```python
from build123d import *

# Parameters (mm, degrees)
CROQUIS1_W              = 30
CROQUIS1_H              = 10
SALIENTE_EXTRUIR1_DEPTH = 2
CORTAR_EXTRUIR2_DEPTH   = 11
CROQUIS3_W              = 11.193843072
CROQUIS3_H              = 1
CROQUIS3_W_2            = 11.806156928
SALIENTE_EXTRUIR3_DEPTH = 1.5
CORTAR_EXTRUIR3_DEPTH   = 11.5
CROQUIS5_W              = 1.4
CROQUIS5_H              = 5
CORTAR_EXTRUIR4_DEPTH   = 10
CROQUIS6_W              = 8
CROQUIS6_H              = 5
SALIENTE_EXTRUIR4_DEPTH = 6
CROQUIS7_W              = 6.2
CROQUIS7_H              = 6
CORTAR_EXTRUIR5_DEPTH   = 11
CORTAR_EXTRUIR6_DEPTH   = 11
REDONDEO1_R             = 1
CROQUIS9_W              = 0.4
CROQUIS9_H              = 1
CORTAR_EXTRUIR7_DEPTH   = 23


with BuildPart() as part:
    # Croquis1 → Saliente-Extruir1 (new body)
    with BuildSketch(Plane.XY):
        Rectangle(CROQUIS1_W, CROQUIS1_H)
    extrude(amount=SALIENTE_EXTRUIR1_DEPTH)

    # Croquis2 → Cortar-Extruir2 (cut)
    with BuildSketch(Plane.XY.offset(2)):
        with BuildLine():
            Line((-13.5, -2.5), (-13.5, 2.5))
            ThreePointArc((-13.5, 2.5), (-12.5, 3.5), (-11.5, 2.5))
            Line((-11.5, 2.5), (-11.5, -2.5))
            ThreePointArc((-11.5, -2.5), (-12.5, -3.5), (-13.5, -2.5))
        make_face()
        with BuildLine():
            Line((11.5, 2.5), (11.5, -2.5))
            ThreePointArc((11.5, -2.5), (12.5, -3.5), (13.5, -2.5))
            Line((13.5, -2.5), (13.5, 2.5))
            ThreePointArc((13.5, 2.5), (12.5, 3.5), (11.5, 2.5))
        make_face()
    extrude(amount=-CORTAR_EXTRUIR2_DEPTH, mode=Mode.SUBTRACT)

    # Croquis3 → Saliente-Extruir3 (add)
    with BuildSketch(Plane(origin=(0, 0, 0), x_dir=(-1, 0, 0), z_dir=(0, 0, -1))):
        with Locations((5.903078464, -1.5)):
            Rectangle(CROQUIS3_W, CROQUIS3_H)
        with Locations((-5.596921536, -1.5)):
            Rectangle(CROQUIS3_W_2, CROQUIS3_H)
    extrude(amount=SALIENTE_EXTRUIR3_DEPTH)

    # Croquis4 → Cortar-Extruir3 (cut)
    with BuildSketch(Plane.XY.offset(2)):
        with BuildLine():
            Line((-13.6, 2.5), (-13.6, -2.5))
            ThreePointArc((-13.6, -2.5), (-12.5, -3.6), (-11.4, -2.5))
            Line((-11.4, -2.5), (-11.4, 2.5))
            ThreePointArc((-11.4, 2.5), (-12.5, 3.6), (-13.6, 2.5))
        make_face()
        with BuildLine():
            Line((11.4, 2.5), (11.4, -2.5))
            ThreePointArc((11.4, -2.5), (12.5, -3.6), (13.6, -2.5))
            Line((13.6, -2.5), (13.6, 2.5))
            ThreePointArc((13.6, 2.5), (12.5, 3.6), (11.4, 2.5))
        make_face()
    extrude(amount=-CORTAR_EXTRUIR3_DEPTH, mode=Mode.SUBTRACT)

    # Croquis5 → Cortar-Extruir4 (cut)
    with BuildSketch(Plane.XY.offset(2)):
        with Locations((-14.3, 0)):
            Rectangle(CROQUIS5_W, CROQUIS5_H)
        with Locations((14.3, 0)):
            Rectangle(CROQUIS5_W, CROQUIS5_H)
    extrude(amount=-CORTAR_EXTRUIR4_DEPTH, mode=Mode.SUBTRACT)

    # Croquis6 → Saliente-Extruir4 (add)
    with BuildSketch(Plane.XY.offset(2)):
        with Locations((0, 2.5)):
            Rectangle(CROQUIS6_W, CROQUIS6_H)
        with Locations((0, -2.5)):
            Rectangle(CROQUIS6_W, CROQUIS6_H)
    extrude(amount=SALIENTE_EXTRUIR4_DEPTH)

    # Croquis7 → Cortar-Extruir5 (cut)
    with BuildSketch(Plane(origin=(0, 5, 0), x_dir=(1, 0, 0), z_dir=(0, 1, 0))):
        with Locations((0, -5)):
            Rectangle(CROQUIS7_W, CROQUIS7_H)
    extrude(amount=-CORTAR_EXTRUIR5_DEPTH, mode=Mode.SUBTRACT)

    # Croquis8 → Cortar-Extruir6 (cut)
    with BuildSketch(Plane.ZY.offset(4)):
        with BuildLine():
            Line((5, -4), (5, 4))
            Line((5, 4), (4, 4))
            ThreePointArc((4, 4), (3.292893219, 3.707106781), (3, 3))
            Line((3, 3), (3, -3))
            ThreePointArc((3, -3), (3.292893219, -3.707106781), (4, -4))
            Line((4, -4), (5, -4))
        make_face()
        with BuildLine():
            Line((6, 4), (5, 4))
            Line((5, 4), (5, -4))
            Line((5, -4), (6, -4))
            ThreePointArc((6, -4), (6.707106781, -3.707106781), (7, -3))
            Line((7, -3), (7, 3))
            ThreePointArc((7, 3), (6.707106781, 3.707106781), (6, 4))
        make_face()
    extrude(amount=-CORTAR_EXTRUIR6_DEPTH, mode=Mode.SUBTRACT)

    # Redondeo1
    redondeo1_edges = [part.edges().sort_by_distance(p)[0] for p in [
        (3.55, 5, 8),
        (-3.55, -5, 8),
        (-3.55, 5, 8),
        (3.55, -5, 8),
    ]]
    fillet(redondeo1_edges, radius=REDONDEO1_R)

    # Croquis9 → Cortar-Extruir7 (cut)
    with BuildSketch(Plane(origin=(11.4, 0, 0), x_dir=(0, 0, -1), z_dir=(1, 0, 0))):
        with Locations((1.3, -1.5)):
            Rectangle(CROQUIS9_W, CROQUIS9_H)
    extrude(amount=-CORTAR_EXTRUIR7_DEPTH, mode=Mode.SUBTRACT)


solid = part.part
```
The model under review builds one solid part; all positions refer to its coordinate system, in mm. A direction names the side the tool comes from. Round coordinates to 2 decimals unless told otherwise and drop trailing zeros. Loops run counter-clockwise (first coordinate to the right, second up) from the corner with the lowest first, then second, coordinate; pieces in that order, holes last. Notation, with made-up numbers: (-6, -10.75) -> (0, -10.75) arc R16 cw to (0, 20.25) -> close; hole circle Ø11 at (84, -39.75). An arc over 180 degrees is marked (long way). Answer as a JSON object with one key per item and string values. Group by question number.
1) We need section C-C on z = 6.5. Write out the cut boundary in (x, y).
2) For line 1 (X direction, y = -2.75, z = 1.75); line 2 (Z direction, x = -9, y = -0.75); line 3 (Y direction, x = 2.75, z = -0.25), list the stretches that pass through material, from the lowest coordinate up. Write a range as [from, to].
3) We need section B-B on y = -0.25. Write out the cut boundary in (x, z).
4) We need section D-D on x = 6. Write out the cut boundary in (y, z).
5) For pin 1 Ø5 at (y, z) = (-2.5, 5.5) entering from +X; pin 2 Ø0.9 at (x, y) = (1.5, -3.5) entering from -Z; pin 3 Ø5 at (y, z) = (2, 5) entering from -X, all flat-tipped, find the tip position at first contact; note any pin that passes through.
6) Mouldability with a two-part tool opening along Z and no side actions: class faces 1 (the face through (-3.6, 4, 5)), 2 (the face through (15, -4, 1)), 3 (the face through (8, 0, 2)) as released by +Z, released by -Z, zero draft, split by the parting line, or undercut.
7) For faces 4 (the face through (-12.5, 3.6, 1)), 5 (the face through (-3.6, -4, 5)), 6 (the face through (-0.2, -1, -0.5)), 7 (the face through (-4, 0.1, 2.3)), list the 3-axis set-ups (+Z, -Z, +X, -X, +Y, -Y) from which the entire face can be reached by the end or side of a thin tool; tool diameter is ignored.
8) We need section A-A on x = -12.5. Write out the cut boundary in (y, z), then the cut area to 3 significant figures.
Result set:
{
 "1": {"outline": "(-4, -5) -> (-3.1, -5) -> (-3.1, -3.87) -> (-4, -3.87) -> close; (-4, 3.87) -> (-3.1, 3.87) -> (-3.1, 5) -> (-4, 5) -> close; (3.1, -5) -> (4, -5) -> (4, -3.87) -> (3.1, -3.87) -> close; (3.1, 3.87) -> (4, 3.87) -> (4, 5) -> (3.1, 5) -> close"},
 "2": {"line 1": "[-15, -13.57], [-11.43, 11.43], [13.57, 15]", "line 2": "[0, 2]", "line 3": "[-2, -1]"},
 "3": {"outline": "(-11.4, 0) -> (11.4, 0) -> (11.4, 2) -> (4, 2) -> (4, 3) -> (3.1, 3) -> (3.1, 2) -> (-3.1, 2) -> (-3.1, 3) -> (-4, 3) -> (-4, 2) -> (-11.4, 2) -> close; (-4, 7) -> (-3.1, 7) -> (-3.1, 8) -> (-4, 8) -> close; (3.1, 7) -> (4, 7) -> (4, 8) -> (3.1, 8) -> close"},
 "4": {"outline": "(-5, 0) -> (-2, 0) -> (-2, -1.1) -> (-1, -1.1) -> (-1, 0) -> (5, 0) -> (5, 2) -> (-5, 2) -> close"},
 "5": {"pin 1": "x = 4", "pin 2": "z = 0", "pin 3": "x = -4"},
 "6": {"face 1": "undercut", "face 2": "zero draft", "face 3": "released by +Z"},
 "7": {"face 4": "+Z, -Z", "face 5": "+X, -X", "face 6": "-Z, +X, -X, +Y", "face 7": "+Z, -X, +Y, -Y"},
 "8": {"outline": "(-5, 0) -> (-3.6, 0) -> (-3.6, 2) -> (-5, 2) -> close; (3.6, 0) -> (5, 0) -> (5, 2) -> (3.6, 2) -> close", "area": "5.60 mm²"}
}
